from build123d import *

# Parameters (mm, degrees)
SKETCH2_W           = 20
SKETCH2_H           = 40
BOSS_EXTRUDE1_DEPTH = 6.5
SKETCH4_W           = 17.997114687
SKETCH4_H           = 38
CUT_EXTRUDE1_DEPTH  = 5.5
CUT_EXTRUDE4_DEPTH  = 1
CUT_EXTRUDE5_DEPTH  = 1
FILLET1_R           = 0.5


with BuildPart() as part:
    # Sketch2 → Boss-Extrude1 (new body)
    with BuildSketch(Plane.XY):
        Rectangle(SKETCH2_W, SKETCH2_H)
    extrude(amount=BOSS_EXTRUDE1_DEPTH)

    # Sketch4 → Cut-Extrude1 (cut)
    with BuildSketch(Plane.XY.offset(6.5)):
        with Locations((-0.001442657, 0)):
            Rectangle(SKETCH4_W, SKETCH4_H)
    extrude(amount=-CUT_EXTRUDE1_DEPTH, mode=Mode.SUBTRACT)

    # Sketch6 → Cut-Extrude4 (cut)
    with BuildSketch(Plane.XZ.offset(20)):
        with BuildLine():
            Line((-5.5, 5), (5.5, 5))
            ThreePointArc((5.5, 5), (7.5, 3), (5.5, 1))
            Line((5.5, 1), (-5.5, 1))
            ThreePointArc((-5.5, 1), (-7.5, 3), (-5.5, 5))
        make_face()
    extrude(amount=-CUT_EXTRUDE4_DEPTH, mode=Mode.SUBTRACT)

    # Sketch8 → Cut-Extrude5 (cut)
    with BuildSketch(Plane(origin=(0, 20, 0), x_dir=(1, 0, 0), z_dir=(0, 1, 0))):
        with BuildLine():
            Line((-3, -1), (3, -1))
            ThreePointArc((3, -1), (4.5, -2.5), (3, -4))
            Line((3, -4), (-3, -4))
            ThreePointArc((-3, -4), (-4.5, -2.5), (-3, -1))
        make_face()
    extrude(amount=-CUT_EXTRUDE5_DEPTH, mode=Mode.SUBTRACT)

    # Fillet1
    fillet1_edges = [part.edges().sort_by_distance(p)[0] for p in [
        (10, -20, 3.25),
        (-10, -20, 3.25),
        (-10, 20, 3.25),
        (10, 20, 3.25),
    ]]
    fillet(fillet1_edges, radius=FILLET1_R)


solid = part.part
CAD build for the part. Positions are in the model's coordinates, mm. A direction names the side the tool comes from. Round coordinates to 2 decimals unless told otherwise and drop trailing zeros. Write each loop counter-clockwise with the first axis right and the second up, starting at its lowest first coordinate (ties: lowest second). Pieces come first, ordered by that corner, then holes. Notation, with made-up numbers: M -18.5,-18 L 33.5,-18 A22 ccw 33.5,-1 Z; hole C 24.5,44 d10. An arc over 180 degrees is marked long. Use a Markdown table: item, result. Add a question column.
1. 3-axis set-ups, long thin cutter, end or side, ignore diameter. For faces 4 (the face through (-9, 0, 4)), 5 (the face through (-4.5, 19.5, 2.5)), 6 (the face through (-7.5, -19.5, 3)), 7 (the face through (-0.1, -20, 5.4)): which of +Z, -Z, +X, -X, +Y, -Y reach the whole face in a straight line?
2. Slice it at D-D on y = 6.5. Give the cut face in (x, z).
3. Drill centre lines: probe 1 along X at (y, z) = (9, 5.75); probe 2 along Y at (x, z) = (-6.75, 5); probe 3 along Z at (x, y) = (6.5, -5). Where is each one in solid material? Low to high.
4. Slice it at C-C on x = 6.5. Give the cut face in (y, z).
5. Slice it at A-A on x = 1.25. Give the cut face in (y, z).
6. Pull direction X, two halves, no side cores. Call faces 1 (the face through (10, 0, 3)), 2 (the face through (8.997, 0, 4)), 3 (the face through (0, 0, 0)): released by +X, released by -X, zero draft, split by the parting line, or undercut.
7. Slice it at B-B on z = 2.5. Give the cut face in (x, y).
8. Flat gauge pin, fed straight in: P1, Ø1.5, axis at x = -6.5, z = 3, coming from the -Y side. Where does the tip first touch, or does it go through?
Reply:
| question | item | result |
|---|---|---|
| 1 | face 4 | +Z |
| 1 | face 5 | +Y, -Y |
| 1 | face 6 | -Y |
| 1 | face 7 | +Z, -Z, +X, -X, -Y |
| 2 | outline | M -10,0 L 10,0 L 10,6.5 L 9,6.5 L 9,1 L -9,1 L -9,6.5 L -10,6.5 Z |
| 3 | probe 1 | x = -10 to -9, 9 to 10 |
| 3 | probe 2 | y = -20 to -19, 19 to 20 |
| 3 | probe 3 | z = 0 to 1 |
| 4 | outline | M -20,0 L 20,0 L 20,6.5 L 19,6.5 L 19,1 L -19,1 L -19,1.27 L -20,1.27 Z; M -20,4.73 L -19,4.73 L -19,6.5 L -20,6.5 Z |
| 5 | outline | M -20,0 L 20,0 L 20,1 L -20,1 Z; M -20,5 L -19,5 L -19,6.5 L -20,6.5 Z; M 19,4 L 20,4 L 20,6.5 L 19,6.5 Z |
| 6 | face 1 | released by +X |
| 6 | face 2 | undercut |
| 6 | face 3 | zero draft |
| 7 | outline | M -10,-19.5 A0.5 ccw -9.5,-20 L -7.44,-20 L -7.44,-19 L -9,-19 L -9,19 L -4.5,19 L -4.5,20 L -9.5,20 A0.5 ccw -10,19.5 Z; M 4.5,19 L 9,19 L 9,-19 L 7.44,-19 L 7.44,-20 L 9.5,-20 A0.5 ccw 10,-19.5 L 10,19.5 A0.5 ccw 9.5,20 L 4.5,20 Z |
| 8 | P1 | stops at y = 19 |
